Autodesk Inventor part; units mm, degrees
ref_plane "YZ Plane" through (0, 0, 0) normal (1, 0, 0) x (0, 1, 0)
ref_plane "XZ Plane" through (0, 0, 0) normal (0, 1, 0) x (-1, 0, 0)
ref_plane "XY Plane" through (0, 0, 0) normal (0, 0, 1) x (1, 0, 0)
sketch "Sketch1" plane through (0, 0, 0) normal (0, 0, 1) x (1, 0, 0)
  circle A0 centre (0, 0) radius 60
  dimension "d0" = 120
extrude "Extrusion1" add sketch "Sketch1" along normal blind 40
sketch "Sketch4" plane through (0, 0, 40) normal (0, 0, 1) x (1, 0, 0)
  line L0 (4.6, 13) -> (39.6, 13)
  line L1 (39.6, 13) -> (39.6, -13)
  line L2 (39.6, -13) -> (4.6, -13)
  line L3 (4.6, -13) -> (4.6, 13)
  line L4 (0, 0) -> (4.6, 0) construction
  dimension "d14" = 35
  dimension "d15" = 26
  dimension "d16" = 4.6
extrude "Extrusion4" cut sketch "Sketch4" against normal blind 30
sketch "Sketch5" plane through (0, 0, 40) normal (0, 0, 1) x (1, 0, 0)
  line L0 (47.6, -17.5) -> (39.6, -17.5)
  line L1 (39.6, -17.5) -> (39.6, 17.5)
  line L2 (39.6, 17.5) -> (47.6, 17.5)
  line L3 (47.6, 17.5) -> (47.6, -17.5)
  line L4 (39.6, 13) -> (39.6, -13)
  point P0 (0, 0)
  point P1 (39.6, 0)
  point P2 (39.6, 0)
  dimension "d19" = 35
  dimension "d20" = 8
extrude "Extrusion5" add sketch "Sketch5" along normal blind 30
sketch "Sketch6" plane through (39.6, -13, 10) normal (-1, 0, 0) x (0, 0, 1)
  circle A0 centre (57, 22) radius 1
  circle A1 centre (57, 4) radius 1
  line L0 (57, 22) -> (57, 4) construction
  line L1 (60, 30.5) -> (60, -4.5) construction
  point P0 (-10, 13)
  point P1 (57, 13)
  point P2 (60, 13)
  dimension "d23" = 18
  dimension "d24" = 2
  dimension "d25" = 2
  dimension "d26" = 3
extrude "Extrusion6" cut sketch "Sketch6" against normal up to surface (8 mm away)
sketch "Sketch7" plane through (0, 0, 0) normal (0, 0, -1) x (-1, 0, 0)
  circle A0 centre (0, 0) radius 39.5
  dimension "d29" = 79
extrude "Extrusion7" cut sketch "Sketch7" against normal blind 5
sketch "Sketch8" plane through (0, 0, 5) normal (0, 0, -1) x (-1, 0, 0)
  circle A0 centre (-33, 0) radius 2
  point P0 (0, 0)
  dimension "d32" = 33
  dimension "d33" = 4
extrude "Extrusion8" cut sketch "Sketch8" against normal blind 5
pattern_circular "Circular Pattern1" count 12 over 360 about axis through (0, 0, 0) along (0, 0, 1) of "Extrusion8"
properties part number "manipulator base"
Build history of the part. All positions in model axes, mm. A direction names the side the tool comes from. Coordinates: 2 decimals unless noted, no trailing zeros. Order: outer loops, then holes, each group sorted by start corner. A loop starts at its lowest first (then second) coordinate and runs counter-clockwise, first axis right, second up. Notation, with made-up numbers: (26, -24) -> (67, -24) arc R33 cw to (67, 7) -> close; hole circle Ø2 at (-34.75, 62). An arc over 180 degrees is marked (long way). One line per item, written item: value.
(1) Slice it at A-A, the plane x = 0. List the corners of the cut face in (y, z).
Checked values:
outline: (-60, 0) -> (-39.5, 0) -> (-39.5, 5) -> (-35, 5) -> (-35, 10) -> (-31, 10) -> (-31, 5) -> (31, 5) -> (31, 10) -> (35, 10) -> (35, 5) -> (39.5, 5) -> (39.5, 0) -> (60, 0) -> (60, 40) -> (-60, 40) -> close
(2) Tool access for faces 1 (the flat face through (44, 17.5, 55)), 2 (the flat face through (44, 0, 70)), 3 (the flat face through (12, -39, 0)), 4 (the flat face through (22, -13, 25)), 5 (the cylindrical face through (0.601, -31.092, 7.465)): list every direction of +Z, -Z, +X, -X, +Y, -Y with a clear straight run to the whole face (end or side of a thin tool).
Checked values:
face 1: +Z, +X, -X, +Y
face 2: +Z, +X, -X, +Y, -Y
face 3: -Z, +X, -X, +Y, -Y
face 4: +Z
face 5: -Z
(3) Mould opens along X. For faces 6 (the flat face through (29, -16, 10)), 7 (the cylindrical face through (30.56, 16.24, 7.46)), 8 (the flat face through (47.6, 0, 55)), 9 (the cylindrical face through (-59.94, -2.64, 19.72)) say: pulls with the +X half, pulls with the -X half, needs draft (parallel to the pull), parting line crosses it, or undercut.
Checked values:
face 6: undercut
face 7: undercut
face 8: pulls with the +X half
face 9: parting line crosses it
(4) Slice it at D-D, the plane y = -33. List the corners of the cut face in (x, z), plus the area to 3 significant figures.
Checked values:
outline: (-50.11, 0) -> (-21.71, 0) -> (-21.71, 5) -> (-2, 5) -> (-2, 10) -> (2, 10) -> (2, 5) -> (21.71, 5) -> (21.71, 0) -> (50.11, 0) -> (50.11, 40) -> (-50.11, 40) -> close
area: 3,770 mm2
(5) Slice it at C-C, the plane x = 33. List the corners of the cut face in (y, z).
Checked values:
outline: (-50.11, 0) -> (-21.71, 0) -> (-21.71, 5) -> (-2, 5) -> (-2, 10) -> (-13, 10) -> (-13, 40) -> (-50.11, 40) -> close; (2, 5) -> (21.71, 5) -> (21.71, 0) -> (50.11, 0) -> (50.11, 40) -> (13, 40) -> (13, 10) -> (2, 10) -> close
(6) Drop flat-ended pins along their axis: pin 1 Ø2 at (x, y) = (16.5, 41) entering from +Z; pin 2 Ø24 at (x, z) = (15.5, 31.5) entering from +Y; pin 3 Ø1 at (x, z) = (15, 28) entering from +Y. Give the stop position or say it passes through.
Checked values:
pin 1: z = 40
pin 2: y = 59.9
pin 3: y = 58.22
(7) Slice it at B-B, the plane z = 35. List the corners of the cut face in (x, y).
Checked values:
outline: circle Ø120 at (0, 0); hole (4.6, -13) -> (39.6, -13) -> (39.6, 13) -> (4.6, 13) -> close
(8) Probe line 1 (Y direction, x = 45, z = 67); line 2 (Y direction, x = -16, z = 6); line 3 (X direction, y = 30, z = 7). List the from-to ranges inside material, lowest first. Write a range as [from, to].
Checked values:
line 1: [-17.5, -10], [-8, 8], [10, 17.5]
line 2: [-57.83, -30.52], [-26.64, 26.64], [30.52, 57.83]
line 3: [-51.96, -17.91], [-15.09, 15.09], [17.91, 51.96]
